```python
from build123d import *

# Parameters (mm, degrees)
SKETCH1_R           = 6.25
BOSS_EXTRUDE1_DEPTH = 3.5
SKETCH2_R           = 4.4
CUT_EXTRUDE1_DEPTH  = 0.5


with BuildPart() as part:
    # Sketch1 → Boss-Extrude1 (new body)
    with BuildSketch(Plane.XY):
        Circle(SKETCH1_R)
    extrude(amount=BOSS_EXTRUDE1_DEPTH)

    # Sketch2 → Cut-Extrude1 (cut)
    with BuildSketch(Plane.XY.offset(3.5)):
        Circle(SKETCH2_R)
    cut_extrude1 = extrude(amount=-CUT_EXTRUDE1_DEPTH, mode=Mode.SUBTRACT)

    # Mirror1: Cut-Extrude1 across plane
    add(cut_extrude1.mirror(Plane.XY.offset(1.75)), mode=Mode.SUBTRACT)


solid = part.part
```
Here's how the part is built. I have some questions about the finished solid (model axes, mm). A direction names the side the tool comes from. Coordinates: 2 decimals unless noted, no trailing zeros. Loops run counter-clockwise (first coordinate to the right, second up) from the corner with the lowest first, then second, coordinate; pieces in that order, holes last. Notation, with made-up numbers: M 68.25,66.25 L 105.25,66.25 A14 cw 105.25,78.25 Z; hole C 56.25,-31.75 d6. An arc over 180 degrees is marked long. One line per item, written item: value.
1. Imagine slicing it at D-D (y = -5). List the corners of the cut face in (x, z) for me, and give its area (4 significant figures).
Geometry says:
outline: M -3.75,0 L 3.75,0 L 3.75,3.5 L -3.75,3.5 Z
area: 26.25 mm2
2. Please list where these lines run through material, in increasing order: probe 1 along Y at (x, z) = (0, 0.1); probe 2 along Z at (x, y) = (2, -3.5); probe 3 along X at (y, z) = (0.5, 0.3).
Geometry says:
probe 1: y = -6.25 to -4.4, 4.4 to 6.25
probe 2: z = 0.5 to 3
probe 3: x = -6.23 to -4.37, 4.37 to 6.23
3. Imagine slicing it at C-C (z = 0.3). List the corners of the cut face in (x, y) for me.
Geometry says:
outline: C 0,0 d12.5; hole C 0,0 d8.8
4. Thinking about a two-plate mould opening in Y: for faces 4 (the cylindrical face through (4.197, 1.322, 0.246)), 5 (the flat face through (-4.3, 1.5, 0)), 6 (the cylindrical face through (5.96, 1.88, 1.73)), which applies, +Y half, -Y half, draft (parallel to the pull), parting line (faces both ways), or undercut?
Geometry says:
face 4: undercut
face 5: draft
face 6: parting line
5. On a 3-axis mill with a long thin cutter (end or side, diameter ignored), from which of +Z, -Z, +X, -X, +Y, -Y can I reach the whole of each face in a straight line? I mean faces 1 (the flat face through (0, 0, 0.5)), 2 (the cylindrical face through (4.197, 1.322, 3.254)), 3 (the flat face through (-4.3, 1.5, 3.5)). Say none if no direction works.
Geometry says:
face 1: -Z
face 2: +Z
face 3: +Z, +X, -X, +Y, -Y
6. Will these pins go through, and if not, where does the flat tip stop? pin 1 Ø1.5 at (x, y) = (5, 1.5) entering from -Z; pin 2 Ø2 at (x, y) = (0, -1) entering from -Z; pin 3 Ø4.5 at (x, y) = (0.5, 0.5) entering from +Z; pin 4 Ø2 at (x, z) = (-2, 1) entering from +Y.
Geometry says:
pin 1: stops at z = 0
pin 2: stops at z = 0.5
pin 3: stops at z = 3
pin 4: stops at y = 6.17
7. Imagine slicing it at A-A (x = 0). List the corners of the cut face in (y, z) for me, and give its area (4 significant figures).
Geometry says:
outline: M -6.25,0 L -4.4,0 L -4.4,0.5 L 4.4,0.5 L 4.4,0 L 6.25,0 L 6.25,3.5 L 4.4,3.5 L 4.4,3 L -4.4,3 L -4.4,3.5 L -6.25,3.5 Z
area: 34.95 mm2
